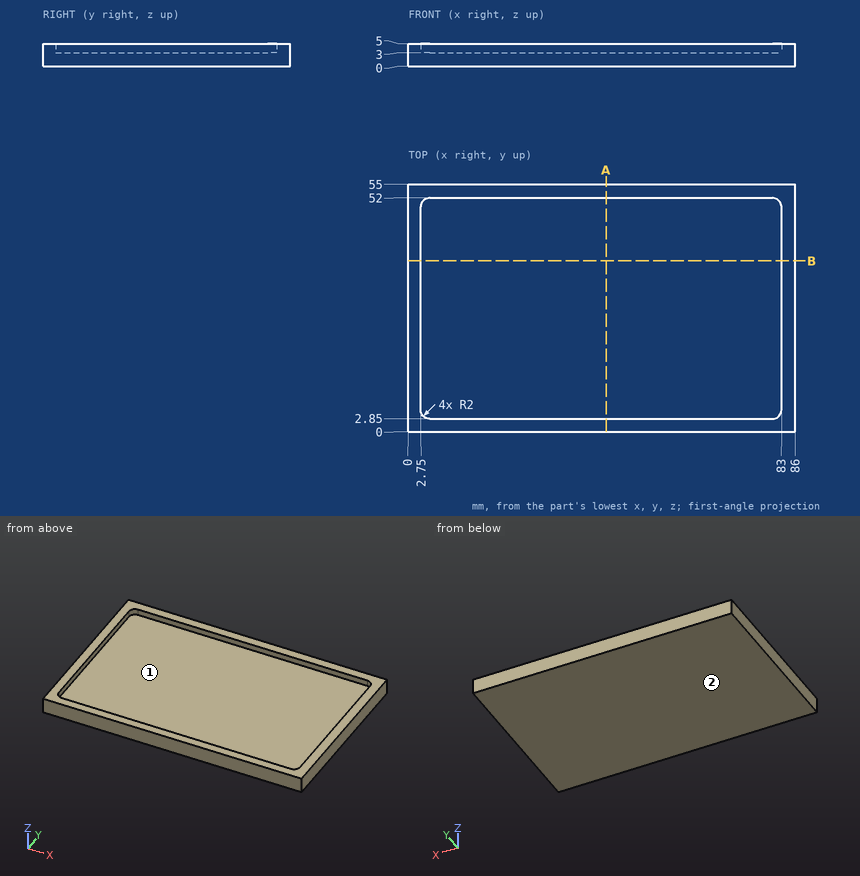
Source: three-view drawing plus pictorial views. Frame: mm from the lowest corner of the part. Round coordinates to 2 decimals unless told otherwise and drop trailing zeros. Order: outer loops, then holes, each group sorted by start corner. A loop starts at its lowest first (then second) coordinate and runs counter-clockwise, first axis right, second up. Notation, with made-up numbers: (74, 88.25) - (123, 88.25) arc R20 cw to (123, 113.25) - close; hole circle Ø2 at (-16, 5). An arc over 180 degrees is marked (long way). Answer in a Markdown table with one row per item.
Item 1: Section query A-A (x = 44). Return the cut outline in (y, z), then the cut area to 3 significant figures.
Model answer:
| item | result |
|---|---|
| outline | (0, 0) - (55, 0) - (55, 5) - (52, 5) - (52, 3) - (2.85, 3) - (2.85, 5) - (0, 5) - close |
| area | 177 mm² |
Item 2: Mould query, pull axis X, two halves, no side actions, for the marked faces 1 and 2. Classes: released by +X, released by -X, zero draft, split by the parting line, or undercut.
Model answer:
| item | result |
|---|---|
| face 1 | undercut |
| face 2 | zero draft |
Item 3: Pin query (flat end, axial travel): pin 1 (1.5 mm diameter, centred on x = 36.5, y = 42.5, fed in from +Z). Return the tip coordinate at first contact, or that it passes through.
Model answer:
| item | result |
|---|---|
| pin 1 | stops at z = 3 |
Item 4: Section query B-B (y = 38). Return the cut outline in (x, z).
Model answer:
| item | result |
|---|---|
| outline | (0, 0) - (86, 0) - (86, 5) - (83, 5) - (83, 3) - (2.75, 3) - (2.75, 5) - (0, 5) - close |
Item 5: Line query: line 1 (Y direction, x = 10.5, z = 4.3); line 2 (X direction, y = 13, z = 4); line 3 (Z direction, x = 79.5, y = 20.5). Output: solid intervals per line, ascending.
Model answer:
| item | result |
|---|---|
| line 1 | y = 0 to 2.85, 52 to 55 |
| line 2 | x = 0 to 2.75, 83 to 86 |
| line 3 | z = 0 to 3 |
